Geometry check sheet. Reference: the model listing, model coordinates, mm. Face numbers are marked on the shaded views. A direction names the side the tool comes from. Round coordinates to 2 decimals unless told otherwise and drop trailing zeros. Write each loop counter-clockwise with the first axis right and the second up, starting at its lowest first coordinate (ties: lowest second). Pieces come first, ordered by that corner, then holes. Notation, with made-up numbers: (-3, -15) -> (5, -15) arc R23 cw to (5, 8) -> close; hole circle Ø7 at (70.25, -39.75). An arc over 180 degrees is marked (long way). One line per question, with ' | ' between items.
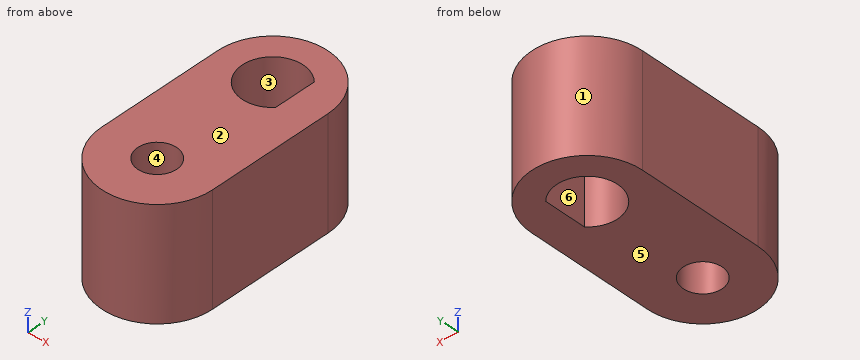
```python
from build123d import *

# Parameters (mm, degrees)
EXTRUDE_2_DEPTH     = 8
SKETCH_1_6_R        = 1.4
CUT_EXTRUDE_2_DEPTH = 8


with BuildPart() as part:
    # 草图1 → 凸台-拉伸2 (new body)
    with BuildSketch(Plane.XY):
        with BuildLine():
            Line((4, 0), (4, -9))
            ThreePointArc((4, -9), (0, -13), (-4, -9))
            Line((-4, -9), (-4, 0))
            ThreePointArc((-4, 0), (0, 4), (4, 0))
        make_face()
    extrude(amount=EXTRUDE_2_DEPTH)

    # 草图1<6> → 切除-拉伸2 (cut)
    with BuildSketch(Plane.XY):
        with BuildLine():
            Line((1.6, -1.509966887), (1.6, 1.509966887))
            ThreePointArc((1.6, 1.509966887), (-2.2, 0), (1.6, -1.509966887))
        make_face()
        with Locations((0, -9)):
            Circle(SKETCH_1_6_R)
    extrude(amount=CUT_EXTRUDE_2_DEPTH, mode=Mode.SUBTRACT)


solid = part.part
```
(1) Sectioned sample at D-D on x = 2.25. Record the cut outline in (y, z), then the cut area to 3 significant figures.
Resolved:
outline: (-12.31, 0) -> (3.31, 0) -> (3.31, 8) -> (-12.31, 8) -> close | area: 125 mm2
(2) Draft check along X on the marked faces 1, 2, 3 and 4. Enter one of: +X half, -X half, draft (parallel to the pull), parting line (faces both ways), or undercut.
Resolved:
face 1: parting line | face 2: draft | face 3: undercut | face 4: undercut
(3) Sectioned sample at A-A on x = 0. Record the cut outline in (y, z), then the cut area to 3 significant figures.
Resolved:
outline: (-13, 0) -> (-10.4, 0) -> (-10.4, 8) -> (-13, 8) -> close; (-7.6, 0) -> (-2.2, 0) -> (-2.2, 8) -> (-7.6, 8) -> close; (2.2, 0) -> (4, 0) -> (4, 8) -> (2.2, 8) -> close | area: 78.4 mm2
(4) Material ranges on line 1 (Y direction, x = 0, z = 6); line 2 (Y direction, x = -1, z = 7.5); line 3 (X direction, y = -2, z = 3), recorded low to high.
Resolved:
line 1: y = -13 to -10.4, -7.6 to -2.2, 2.2 to 4 | line 2: y = -12.87 to -9.98, -8.02 to -1.96, 1.96 to 3.87 | line 3: x = -4 to -0.92, 0.92 to 4
(5) Go/stop test with flat-tipped pins: pin 1 (1.5 mm diameter, centred on x = 1, z = 3, fed in from +Y); pin 2 (2 mm diameter, centred on x = -2.5, z = 3.5, fed in from +Y). Record where each tip stops, or that it passes through.
Resolved:
pin 1: stops at y = 3.99 | pin 2: stops at y = 3.71
(6) Access from +Z, -Z, +X, -X, +Y, -Y to the whole of each face (thin tool, end or side, straight path). Record for the marked faces 5 and 6.
Resolved:
face 5: -Z, +X, -X, +Y, -Y | face 6: +Z, -Z
(7) Sectioned sample at C-C on y = -10. Record the cut outline in (x, z), then the cut area to 3 significant figures.
Resolved:
outline: (-3.87, 0) -> (-0.98, 0) -> (-0.98, 8) -> (-3.87, 8) -> close; (0.98, 0) -> (3.87, 0) -> (3.87, 8) -> (0.98, 8) -> close | area: 46.3 mm2
(8) Sectioned sample at B-B on z = 1.25. Record the cut outline in (x, y).
Resolved:
outline: (-4, -9) arc R4 ccw to (4, -9) -> (4, 0) arc R4 ccw to (-4, 0) -> close; hole circle Ø2.8 at (0, -9); hole (1.6, -1.51) -> (1.6, 1.51) arc R2.2 ccw (long way) to start
